Can you work these out from the model? Positions are in its coordinate system, mm. Face numbers are marked on the shaded views. Round coordinates to 2 decimals unless told otherwise and drop trailing zeros. Order: outer loops, then holes, each group sorted by start corner. A loop starts at its lowest first (then second) coordinate and runs counter-clockwise, first axis right, second up.
from build123d import *

# Parameters (mm, degrees)
F0_R     = 10
F0_R_2   = 7.5
F1_DEPTH = 45
F2_DEPTH = 5
F3_R     = 10
F3_R_2   = 8.4
F4_DEPTH = 30
F5_SIZE  = 2
F6_W     = 5
F6_H     = 16.3043601838
F7_DEPTH = 35
F8_R     = 2
F9_R     = 1


with BuildPart() as f1:
    # F0 (on Top) → F1 (new body)
    with BuildSketch(Plane.XY):
        Circle(F0_R)
        Circle(F0_R_2, mode=Mode.SUBTRACT)
    extrude(amount=F1_DEPTH)

    # F0 (on Top) → F2 (join)
    with BuildSketch(Plane.XY):
        Circle(F0_R)
        Circle(F0_R_2, mode=Mode.SUBTRACT)
        Circle(F0_R_2)
    extrude(amount=F2_DEPTH)

    # F3 (on Top) + F0 (on Top) → F4 (join)
    with BuildSketch(Plane.XY):
        Circle(F3_R)
        Circle(F3_R_2, mode=Mode.SUBTRACT)
    with BuildSketch(Plane.XY):
        Circle(F0_R_2)
    extrude(amount=-F4_DEPTH)

    # F5
    f5_edges = [f1.edges().sort_by_distance(p)[0] for p in [
        (-7.5, 0, -30),
    ]]
    chamfer(f5_edges, length=F5_SIZE)

    # F6 (on face) → F7 (cut)
    with BuildSketch(Plane.XY.offset(45)):
        with Locations((0, 8.1521800919)):
            Rectangle(F6_W, F6_H)
    extrude(amount=-F7_DEPTH, mode=Mode.SUBTRACT)

    # F8
    f8_edges = [f1.edges().sort_by_distance(p)[0] for p in [
        (2.5, 8.376763, 10),
        (-2.5, 8.376763, 10),
    ]]
    fillet(f8_edges, radius=F8_R)

    # F9
    f9_edges = [f1.edges().sort_by_distance(p)[0] for p in [
        (-6.123724, -7.905694, 45),
        (7.905694, 6.123724, 45),
        (-4.330127, -6.123724, 45),
        (6.123724, 4.330127, 45),
    ]]
    fillet(f9_edges, radius=F9_R)


solid = f1.part
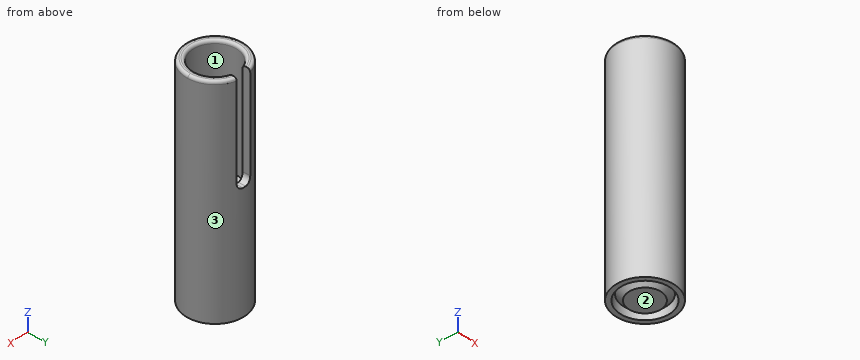
(1) Please list where these lines run through material, in increasing order: probe 1 along Y at (x, z) = (0, -9.25); probe 2 along X at (y, z) = (0, 31); probe 3 along X at (y, z) = (4.25, -15).
(2) I'm going to push flat-ended pins straight in: pin 1 Ø3 at (y, z) = (8, 21.5) entering from +X; pin 2 Ø7.5 at (x, y) = (3, -1.5) entering from +Z; pin 3 Ø12 at (y, z) = (6.5, -5) entering from +X. Where does each tip first touch, or does it pass through?
(3) I want a section at A-A, the plane z = -1.5. List the corners of the cut face in (x, y) for me.
(4) If we mould it in two halves opening along X, with no side actions, what happens to the marked faces 1, 2 and 3? For each: pulls with the +X half, pulls with the -X half, needs draft (parallel to the pull), parting line crosses it, or undercut.
(5) I want a section at B-B, the plane z = 28. List the corners of the cut face in (x, y) for me.
Ans:
1. probe 1: y = -10 to -8.4, -7.5 to 7.5, 8.4 to 10
1. probe 2: x = -10 to -7.5, 7.5 to 10
1. probe 3: x = -9.05 to -7.25, -6.18 to 6.18, 7.25 to 9.05
2. pin 1: stops at x = 7.6
2. pin 2: stops at z = 5
2. pin 3: stops at x = 9.99
3. outline: circle Ø20 at (0, 0); circle Ø15 at (0, 0); hole circle Ø16.8 at (0, 0)
4. face 1: undercut
4. face 2: needs draft
4. face 3: parting line crosses it
5. outline: (-2.5, 7.07) - (-2.5, 9.68) arc R10 ccw (long way) to (2.5, 9.68) - (2.5, 7.07) arc R7.5 cw (long way) to start
